Part model, mm, in its own coordinate system. A direction names the side the tool comes from. Give positions to 0.01 mm unless a question says otherwise; leave off trailing zeros. Order: outer loops, then holes, each group sorted by start corner. A loop starts at its lowest first (then second) coordinate and runs counter-clockwise, first axis right, second up. Notation, with made-up numbers: (4, -40) -> (62, -40) arc R27 cw to (62, -5) -> close; hole circle Ø8 at (-19.75, 1). An arc over 180 degrees is marked (long way). Write item = value, one per line. Start each with the question number.
Item 1: Band-saw the part on C-C on z = 2. Count the separate pieces of the cut face and the enclosed holes in it, plus the area to 3 significant figures.
Item 2: Tool access for faces 5 (the face through (33, 100, 3)), 6 (the face through (48, 4, 3)): list every direction of +Z, -Z, +X, -X, +Y, -Y with a clear straight run to the whole face (end or side of a thin tool).
Item 3: Band-saw the part on A-A on y = -21. Write the cut outline in (x, z), plus the area to 3 significant figures.
Item 4: Drill centre lines: line 1 along X through (y, z) = (152, 4.05); line 2 along Y through (x, z) = (-3, 2.9); line 3 along Y through (x, z) = (26.5, 2.6). Where is each one in solid material? Low to high.
Item 5: Band-saw the part on B-B on x = 16. Write the cut outline in (y, z), plus the area to 3 significant figures.
Item 6: Pull direction Y, two halves, no side cores. Call faces 1 (the face through (0, 141, 3)), 2 (the face through (-36, 7, 0)), 3 (the face through (-1, -144, 3)), 4 (the face through (0, -129, 3)): +Y half, -Y half, draft (parallel to the pull), parting line (faces both ways), or undercut.
```python
from build123d import *

# Parameters (mm, degrees)
SKETCH1_W           = 96
SKETCH1_H           = 300
SKETCH1_W_2         = 66
SKETCH1_H_2         = 80
BOSS_EXTRUDE1_DEPTH = 6
SKETCH3_R           = 1
CUT_EXTRUDE6_DEPTH  = 10
SKETCH5_R           = 1
CUT_EXTRUDE9_DEPTH  = 10
SKETCH7_R           = 1
CUT_EXTRUDE10_DEPTH = 10


with BuildPart() as part:
    # Sketch1 → Boss-Extrude1 (new body)
    with BuildSketch(Plane.XY):
        with Locations((0, 6)):
            Rectangle(SKETCH1_W, SKETCH1_H)
        with Locations((0, 101)):
            Rectangle(SKETCH1_W_2, SKETCH1_H_2, mode=Mode.SUBTRACT)
        with Locations((0, -89)):
            Rectangle(SKETCH1_W_2, SKETCH1_H_2, mode=Mode.SUBTRACT)
        with Locations((0, 6)):
            Rectangle(SKETCH1_W_2, SKETCH1_H_2, mode=Mode.SUBTRACT)
    extrude(amount=BOSS_EXTRUDE1_DEPTH)

    # Sketch3 → Cut-Extrude6 (cut)
    with BuildSketch(Plane.XY.offset(6)):
        with Locations((-39, 126)):
            Circle(SKETCH3_R)
        with Locations((-39, -4)):
            Circle(SKETCH3_R)
        with Locations((-39, 66)):
            Circle(SKETCH3_R)
        with Locations((-39, -64)):
            Circle(SKETCH3_R)
        with Locations(Location((39, -64, 0), (0, 0, 180))):
            Circle(SKETCH3_R)
        with Locations(Location((39, -4, 0), (0, 0, 180))):
            Circle(SKETCH3_R)
        with Locations(Location((39, 66, 0), (0, 0, 180))):
            Circle(SKETCH3_R)
        with Locations(Location((39, 126, 0), (0, 0, 180))):
            Circle(SKETCH3_R)
    extrude(amount=-CUT_EXTRUDE6_DEPTH, mode=Mode.SUBTRACT)

    # Sketch5 → Cut-Extrude9 (cut)
    with BuildSketch(Plane.XY.offset(6)):
        with Locations((-26.5, -134.5)):
            Circle(SKETCH5_R)
        with Locations((26.5, -134.5)):
            Circle(SKETCH5_R)
        with Locations((-26.5, 145.5)):
            Circle(SKETCH5_R)
        with Locations((26.5, 145.5)):
            Circle(SKETCH5_R)
    extrude(amount=-CUT_EXTRUDE9_DEPTH, mode=Mode.SUBTRACT)

    # Sketch7 → Cut-Extrude10 (cut)
    with BuildSketch(Plane.XY.offset(6)):
        with Locations((45, -140)):
            Circle(SKETCH7_R)
        with Locations((-45, -140)):
            Circle(SKETCH7_R)
        with Locations((45, 152)):
            Circle(SKETCH7_R)
        with Locations((-45, 152)):
            Circle(SKETCH7_R)
        with Locations((45, 6)):
            Circle(SKETCH7_R)
        with Locations((-45, 6)):
            Circle(SKETCH7_R)
    extrude(amount=-CUT_EXTRUDE10_DEPTH, mode=Mode.SUBTRACT)


solid = part.part
```
Values found:
q1.separate_pieces = 1
q1.enclosed_holes = 21
q1.area = 12,900 mm^2
q2.face_5 = +Z, -Z
q2.face_6 = +Z, -Z, +X, +Y, -Y
q3.outline = (-48, 0) -> (-33, 0) -> (-33, 6) -> (-48, 6) -> close; (33, 0) -> (48, 0) -> (48, 6) -> (33, 6) -> close
q3.area = 180 mm^2
q4.line_1 = -48 to -46, -44 to 44, 46 to 48
q4.line_2 = -144 to -129, -49 to -34, 46 to 61, 141 to 156
q4.line_3 = -144 to -135.5, -133.5 to -129, -49 to -34, 46 to 61, 141 to 144.5, 146.5 to 156
q5.outline = (-144, 0) -> (-129, 0) -> (-129, 6) -> (-144, 6) -> close; (-49, 0) -> (-34, 0) -> (-34, 6) -> (-49, 6) -> close; (46, 0) -> (61, 0) -> (61, 6) -> (46, 6) -> close; (141, 0) -> (156, 0) -> (156, 6) -> (141, 6) -> close
q5.area = 360 mm^2
q6.face_1 = undercut
q6.face_2 = draft
q6.face_3 = -Y half
q6.face_4 = undercut
